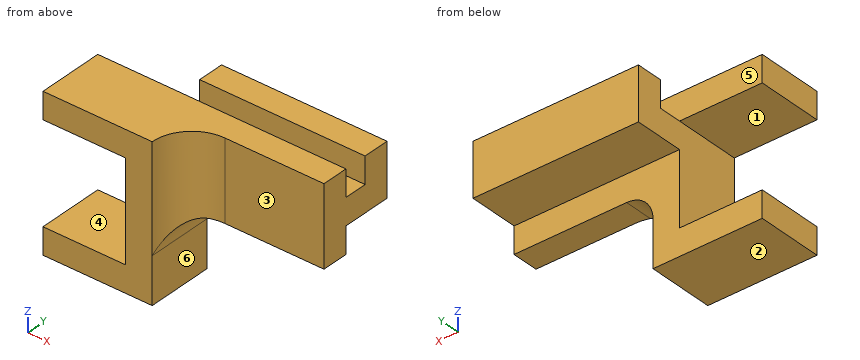
Autodesk Inventor part; units mm, degrees
sketch "Sketch2" plane through (0, 0, 0) normal (1, 0, 0) x (0, 1, 0)
  line L0 (0, -7.6) -> (0, -1.6)
  line L1 (0, 3.44) -> (0, -9.44)
  line L2 (-5.4, 0) -> (4.4, 0)
  line L3 (0, -1.6) -> (3, -1.6)
  line L4 (3, -1.6) -> (3, 1.6)
  line L5 (3, 1.6) -> (1.4, 1.6)
  line L6 (1.4, 1.6) -> (1.4, 0)
  line L7 (1.4, 0) -> (0, 0)
  line L8 (0, 0) -> (0, 1.6)
  line L9 (0, 1.6) -> (-4, 1.6)
  line L10 (-4, 1.6) -> (-4, 1.6)
  line L11 (-4, 1.6) -> (-4, -7.6)
  line L12 (-4, -7.6) -> (0, -7.6)
  point P0 (0, 0)
  dimension "d1" = 6
  dimension "d2" = 3
  dimension "d3" = 3.2
  dimension "d4" = 1.6
  dimension "d6" = 4
  dimension "d7" = 1.6
  dimension "d8" = 1.4
  dimension "d12" = 1.6
extrude "Extrusion1" add sketch "Sketch2" along normal mid plane 10
sketch "Sketch3" plane through (0, 0, 0) normal (0, 0, 1) x (1, 0, 0)
  line L0 (5, 0) -> (5, 3)
  line L1 (5, 0) -> (5, -1.6)
  line L2 (5, -4) -> (5, 0)
  line L3 (-5, -4) -> (5, -4)
  line L4 (-3.4, -4) -> (-3.4, -4)
  line L5 (-5, 0) -> (-5, -4)
  line L6 (5, -1.6) -> (-1, -1.6)
  arc A0 (-1, -1.6) -> (-3.4, -4) centre (-1, -4) ccw
  point P0 (0, 0)
  point P1 (-3.4, -4)
  dimension "d14" = 1.6
  dimension "d15" = 1.6
  dimension "d17" = 2.4
extrude "Extrusion2" cut sketch "Sketch3" along normal through all both and the other way through all
sketch "Sketch4" plane through (-5, 0, 0) normal (-1, 0, 0) x (0, 0, 1)
  line L0 (1.6, 0) -> (0, 0)
  line L1 (-7.6, -4) -> (1.6, -4)
  line L2 (1.6, 0) -> (0, 0)
  line L3 (0, 0) -> (0, -4)
  line L4 (0, -4) -> (1.6, -4)
  line L5 (1.6, -4) -> (1.6, 0)
  line L6 (-1.6, 0) -> (-7.6, 0)
  line L7 (-7.6, 0) -> (-6, 0)
  line L8 (-6, 0) -> (-6, -4)
  line L9 (-6, -4) -> (-7.6, -4)
  line L10 (-7.6, -4) -> (-7.6, 0)
  point P0 (-7.6, -4)
  point P1 (-6, 0)
  point P2 (0, 0)
  dimension "d20" = 1.6
  dimension "d21" = 1.6
extrude "Extrusion3" add sketch "Sketch4" along normal blind 5
sketch "Sketch6" plane through (-5, 0, -1.6) normal (0, 1, 0) x (1, 0, 0)
  line L0 (-5, 6) -> (10, 6)
  line L1 (1.6, 6) -> (1.6, 3.2)
  line L2 (0, 0) -> (0, 4.4)
  line L3 (10, 6) -> (10, 0)
  line L4 (10, 1.6) -> (3.2, 1.6)
  line L5 (0, 0) -> (10, 0)
  arc A0 (1.6, 3.2) -> (3.2, 1.6) centre (3.2, 3.2) ccw
  point P0 (5, -1.6)
  point P1 (0, 6)
  dimension "d24" = 1.6
  dimension "d25" = 1.6
  dimension "d26" = 1.6
extrude "Extrusion4" cut sketch "Sketch6" along normal through all both and the other way through all
properties part number "Hanging_Wall"
Build history of the part. All positions in model axes, mm. Face numbers are marked on the shaded views. A direction names the side the tool comes from. Round coordinates to 2 decimals unless told otherwise and drop trailing zeros. Order: outer loops, then holes, each group sorted by start corner. A loop starts at its lowest first (then second) coordinate and runs counter-clockwise, first axis right, second up. Notation, with made-up numbers: (-34, 73) -> (12, 73) arc R25 cw to (12, 98) -> close; hole circle Ø3 at (57.25, 15). An arc over 180 degrees is marked (long way). Answer in a Markdown table with one row per item.
1) Band-saw the part on A-A on z = 0.5. Give the cut face in (x, y), and give its area (3 significant figures).
Values:
| item | result |
|---|---|
| outline | (-10, -4) -> (-3.4, -4) arc R2.4 cw to (-1, -1.6) -> (5, -1.6) -> (5, 0) -> (-10, 0) -> close; (-5, 1.4) -> (5, 1.4) -> (5, 3) -> (-5, 3) -> close |
| area | 57.1 mm2 |
2) Band-saw the part on D-D on x = 1. Give the cut face in (y, z), and give its area (3 significant figures).
Values:
| item | result |
|---|---|
| outline | (-1.6, -3.2) -> (0, -3.2) -> (0, -1.6) -> (3, -1.6) -> (3, 1.6) -> (1.4, 1.6) -> (1.4, 0) -> (0, 0) -> (0, 1.6) -> (-1.6, 1.6) -> close |
| area | 15.0 mm2 |
3) Band-saw the part on B-B on x = -8.75. Give the cut face in (y, z), and give its area (3 significant figures).
Values:
| item | result |
|---|---|
| outline | (-4, -7.6) -> (0, -7.6) -> (0, -6) -> (-4, -6) -> close; (-4, 0) -> (0, 0) -> (0, 1.6) -> (-4, 1.6) -> close |
| area | 12.8 mm2 |
4) Mould opens along Z. For the marked faces 1, 2 and 3 say: released by +Z, released by -Z, zero draft, split by the parting line, or undercut.
Values:
| item | result |
|---|---|
| face 1 | undercut |
| face 2 | released by -Z |
| face 3 | zero draft |
5) Which spindle directions (+Z, -Z, +X, -X, +Y, -Y) get a long thin tool onto all of the face, cutting with end or side? Do the marked faces 4, 5 and 6. Say none if no direction does.
Values:
| item | result |
|---|---|
| face 4 | -X, +Y, -Y |
| face 5 | +Z, +X, -X |
| face 6 | -Z, +X, +Y, -Y |
6) Band-saw the part on C-C on y = -1. Give the cut face in (x, z), and give its area (3 significant figures).
Values:
| item | result |
|---|---|
| outline | (-10, -7.6) -> (-3.4, -7.6) -> (-3.4, -4.8) arc R1.6 cw to (-1.8, -3.2) -> (5, -3.2) -> (5, 1.6) -> (-10, 1.6) -> (-10, 0) -> (-5, 0) -> (-5, -6) -> (-10, -6) -> close |
| area | 71.6 mm2 |
7) Pin check, flat tips, straight feed: P1, Ø0.8, axis at y = -2, z = -6, coming from the +X side; P2, Ø1.4, axis at x = 3, z = -2, coming from the -Y side; P3, Ø1.3, axis at x = -1.5, z = 1, coming from the -Y side; P4, Ø1.5, axis at x = 2.5, y = -2.5, coming from the -Z side. Stop position of each tip, or through.
Values:
| item | result |
|---|---|
| P1 | x = -3.4 |
| P2 | y = -1.6 |
| P3 | y = -1.89 |
| P4 | through |
8) Wall check: L1, parallel to Y at x = 1.75, z = 0.25; L2, parallel to X at y = -1.75, z = -7; L3, parallel to Y at x = -7.25, z = 1.25. Give the ranges that are in metal, low to high.
Values:
| item | result |
|---|---|
| L1 | -1.6 to 0, 1.4 to 3 |
| L2 | -10 to -3.4 |
| L3 | -4 to 0 |
